Input: part model. Units: mm. Frame: model coordinates. Give positions to 0.01 mm unless a question says otherwise; leave off trailing zeros. Loops run counter-clockwise (first coordinate to the right, second up) from the corner with the lowest first, then second, coordinate; pieces in that order, holes last. Notation, with made-up numbers: (38, 46.5) -> (97, 46.5) arc R14 ccw to (97, 60.5) -> close; hole circle Ø3 at (-6.5, 67.5). An arc over 180 degrees is marked (long way). Answer as a JSON object with one key per item and string values. Group by question number.
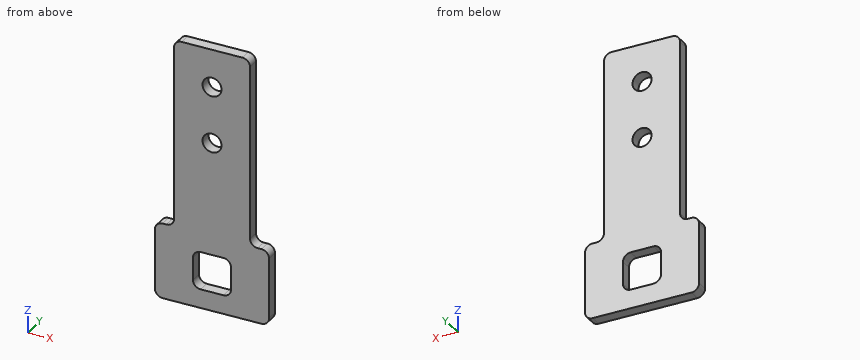
```python
from build123d import *

# Parameters (mm, degrees)
SKETCH_1_R      = 2.5
EXTRUDE_1_DEPTH = 3


with BuildPart() as part:
    # 草图1 → 凸台-拉伸1 (new body)
    with BuildSketch(Plane(origin=(0, 0, 0), x_dir=(1, 0, 0), z_dir=(0, 1, 0))):
        with BuildLine():
            Line((22, 50), (23, 50))
            ThreePointArc((23, 50), (24.414213562, 50.585786438), (25, 52))
            Line((25, 52), (25, 68))
            ThreePointArc((25, 68), (24.414213562, 69.414213562), (23, 70))
            Line((23, 70), (-3, 70))
            ThreePointArc((-3, 70), (-4.414213562, 69.414213562), (-5, 68))
            Line((-5, 68), (-5, 52))
            ThreePointArc((-5, 52), (-4.414213562, 50.585786438), (-3, 50))
            Line((-3, 50), (-2, 50))
            ThreePointArc((-2, 50), (-0.585786438, 49.414213562), (0, 48))
            Line((0, 48), (0, 2))
            ThreePointArc((0, 2), (0.585786438, 0.585786438), (2, 0))
            Line((2, 0), (18, 0))
            ThreePointArc((18, 0), (19.414213562, 0.585786438), (20, 2))
            Line((20, 2), (20, 48))
            ThreePointArc((20, 48), (20.585786438, 49.414213562), (22, 50))
        make_face()
        with Locations(Location((10, 25, 0), (0, 0, 270))):
            Circle(SKETCH_1_R, mode=Mode.SUBTRACT)
        with Locations(Location((10, 10, 0), (0, 0, 270))):
            Circle(SKETCH_1_R, mode=Mode.SUBTRACT)
        with BuildLine():
            Line((7, 65), (13, 65))
            ThreePointArc((13, 65), (14.414213562, 64.414213562), (15, 63))
            Line((15, 63), (15, 57))
            ThreePointArc((15, 57), (14.414213562, 55.585786438), (13, 55))
            Line((13, 55), (7, 55))
            ThreePointArc((7, 55), (5.585786438, 55.585786438), (5, 57))
            Line((5, 57), (5, 63))
            ThreePointArc((5, 63), (5.585786438, 64.414213562), (7, 65))
        make_face(mode=Mode.SUBTRACT)
    extrude(amount=-EXTRUDE_1_DEPTH)


solid = part.part
```
Q1. Section C-C on x = 10. Return the cut outline in (y, z).
Q2. Ray query, probe 1 along X at (y, z) = (-1.3, -10); probe 2 along Z at (x, y) = (13, -0.8); probe 3 along X at (y, z) = (-0.95, -63). Return the intervals inside material, ascending.
Q3. Pin query (flat end, axial travel): pin 1 Ø0.8 at (x, y) = (22.5, -2) entering from +Z; pin 2 Ø0.9 at (y, z) = (-1.5, -25) entering from -X. Return the tip coordinate at first contact, or that it passes through.
Q4. Section A-A on y = -0.45. Return the cut outline in (x, z), then the cut area to 3 significant figures.
Q5. Section B-B on z = -10. Return the cut outline in (x, y), then the cut area to 3 significant figures.
Numbers:
{
 "1": {"outline": "(-3, -70) -> (0, -70) -> (0, -65) -> (-3, -65) -> close; (-3, -55) -> (0, -55) -> (0, -27.5) -> (-3, -27.5) -> close; (-3, -22.5) -> (0, -22.5) -> (0, -12.5) -> (-3, -12.5) -> close; (-3, -7.5) -> (0, -7.5) -> (0, 0) -> (-3, 0) -> close"},
 "2": {"probe 1": "x = 0 to 7.5, 12.5 to 20", "probe 2": "z = -70 to -65, -55 to 0", "probe 3": "x = -5 to 5, 15 to 25"},
 "3": {"pin 1": "stops at z = -50", "pin 2": "stops at x = 0"},
 "4": {"outline": "(-5, -68) arc R2 ccw to (-3, -70) -> (23, -70) arc R2 ccw to (25, -68) -> (25, -52) arc R2 ccw to (23, -50) -> (22, -50) arc R2 cw to (20, -48) -> (20, -2) arc R2 ccw to (18, 0) -> (2, 0) arc R2 ccw to (0, -2) -> (0, -48) arc R2 cw to (-2, -50) -> (-3, -50) arc R2 ccw to (-5, -52) -> close; hole (5, -63) arc R2 ccw to (7, -65) -> (13, -65) arc R2 ccw to (15, -63) -> (15, -57) arc R2 ccw to (13, -55) -> (7, -55) arc R2 ccw to (5, -57) -> close; hole circle Ø5 at (10, -25); hole circle Ø5 at (10, -10)", "area": "1,460 mm²"},
 "5": {"outline": "(0, -3) -> (7.5, -3) -> (7.5, 0) -> (0, 0) -> close; (12.5, -3) -> (20, -3) -> (20, 0) -> (12.5, 0) -> close", "area": "45.0 mm²"}
}
